```python
from build123d import *

# Parameters (mm, degrees)
SKETCH1_R           = 3.38
SKETCH1_W           = 189.625170906
SKETCH1_H           = 189.625170906
BOSS_EXTRUDE1_DEPTH = 9.525


with BuildPart() as part:
    # Sketch1 → Boss-Extrude1 (new body)
    with BuildSketch(Plane.XY):
        Polygon((16.997849507, 0), (0, -16.997849507), (0, -195.854150493), (16.997849507, -212.852), (195.854150493, -212.852), (212.852, -195.854150493), (212.852, -16.997849507), (195.854150493, 0), align=None)
        with Locations(Location((30.226, -208.026, 0), (0, 0, 180))):
            Circle(SKETCH1_R, mode=Mode.SUBTRACT)
        with Locations(Location((4.826, -182.626, 0), (0, 0, 180))):
            Circle(SKETCH1_R, mode=Mode.SUBTRACT)
        with Locations(Location((55.626, -208.026, 0), (0, 0, 180))):
            Circle(SKETCH1_R, mode=Mode.SUBTRACT)
        with Locations(Location((81.026, -208.026, 0), (0, 0, 180))):
            Circle(SKETCH1_R, mode=Mode.SUBTRACT)
        with Locations(Location((4.826, -157.226, 0), (0, 0, 180))):
            Circle(SKETCH1_R, mode=Mode.SUBTRACT)
        with Locations(Location((4.826, -131.826, 0), (0, 0, 180))):
            Circle(SKETCH1_R, mode=Mode.SUBTRACT)
        with Locations(Location((4.826, -106.426, 0), (0, 0, 180))):
            Circle(SKETCH1_R, mode=Mode.SUBTRACT)
        with Locations(Location((106.426, -208.026, 0), (0, 0, 180))):
            Circle(SKETCH1_R, mode=Mode.SUBTRACT)
        with Locations(Location((131.826, -208.026, 0), (0, 0, 180))):
            Circle(SKETCH1_R, mode=Mode.SUBTRACT)
        with Locations(Location((157.226, -208.026, 0), (0, 0, 180))):
            Circle(SKETCH1_R, mode=Mode.SUBTRACT)
        with Locations(Location((182.626, -208.026, 0), (0, 0, 180))):
            Circle(SKETCH1_R, mode=Mode.SUBTRACT)
        with Locations(Location((208.026, -182.626, 0), (0, 0, 180))):
            Circle(SKETCH1_R, mode=Mode.SUBTRACT)
        with Locations(Location((208.026, -157.226, 0), (0, 0, 180))):
            Circle(SKETCH1_R, mode=Mode.SUBTRACT)
        with Locations(Location((208.026, -131.826, 0), (0, 0, 180))):
            Circle(SKETCH1_R, mode=Mode.SUBTRACT)
        with Locations(Location((4.826, -81.026, 0), (0, 0, 180))):
            Circle(SKETCH1_R, mode=Mode.SUBTRACT)
        with Locations(Location((4.826, -55.626, 0), (0, 0, 180))):
            Circle(SKETCH1_R, mode=Mode.SUBTRACT)
        with Locations(Location((4.826, -30.226, 0), (0, 0, 180))):
            Circle(SKETCH1_R, mode=Mode.SUBTRACT)
        with Locations(Location((30.226, -4.826, 0), (0, 0, 180))):
            Circle(SKETCH1_R, mode=Mode.SUBTRACT)
        with Locations(Location((55.626, -4.826, 0), (0, 0, 180))):
            Circle(SKETCH1_R, mode=Mode.SUBTRACT)
        with Locations(Location((81.026, -4.826, 0), (0, 0, 180))):
            Circle(SKETCH1_R, mode=Mode.SUBTRACT)
        with Locations((106.426, -106.426)):
            Rectangle(SKETCH1_W, SKETCH1_H, mode=Mode.SUBTRACT)
        with Locations(Location((208.026, -106.426, 0), (0, 0, 180))):
            Circle(SKETCH1_R, mode=Mode.SUBTRACT)
        with Locations(Location((208.026, -81.026, 0), (0, 0, 180))):
            Circle(SKETCH1_R, mode=Mode.SUBTRACT)
        with Locations(Location((208.026, -55.626, 0), (0, 0, 180))):
            Circle(SKETCH1_R, mode=Mode.SUBTRACT)
        with Locations(Location((106.426, -4.826, 0), (0, 0, 180))):
            Circle(SKETCH1_R, mode=Mode.SUBTRACT)
        with Locations(Location((131.826, -4.826, 0), (0, 0, 180))):
            Circle(SKETCH1_R, mode=Mode.SUBTRACT)
        with Locations(Location((157.226, -4.826, 0), (0, 0, 180))):
            Circle(SKETCH1_R, mode=Mode.SUBTRACT)
        with Locations(Location((208.026, -30.226, 0), (0, 0, 180))):
            Circle(SKETCH1_R, mode=Mode.SUBTRACT)
        with Locations(Location((182.626, -4.826, 0), (0, 0, 180))):
            Circle(SKETCH1_R, mode=Mode.SUBTRACT)
    extrude(amount=BOSS_EXTRUDE1_DEPTH)


solid = part.part
```
Can you work these out from the model? Positions are in its coordinate system, mm. A direction names the side the tool comes from. Round coordinates to 2 decimals unless told otherwise and drop trailing zeros. Loops run counter-clockwise (first coordinate to the right, second up) from the corner with the lowest first, then second, coordinate; pieces in that order, holes last.
Item 1: Will these pins go through, and if not, where does the flat tip stop? pin 1 Ø6 at (x, y) = (55.626, -208.026) entering from -Z; pin 2 Ø8 at (x, y) = (55.626, -4.826) entering from -Z.
Item 2: Suppose I cut it at C-C, the plane z = 4.75. State how many separate pieces and enclosed holes the cut face has, then the cut area to 3 significant figures.
Item 3: Which directions (+Z, -Z, +X, -X, +Y, -Y) give clear straight access to the entire face, cutting with the end or side of a thin tool? Please do faces 1 (the flat face through (11.613, -108, 5)), 2 (the flat face through (212.852, -108, 5)).
Item 4: Suppose I cut it at A-A, the plane y = -174. Write out the boundary of the cut face in (x, z) (3 decimals), then the cut area to 3 significant figures.
Item 5: Please list where these lines run through material, in increasing order: L1, parallel to Y at x = 106, z = 2.5; L2, parallel to Y at x = 60.5, z = 2.25; L3, parallel to X at y = -20, z = 5.5.
Item 6: If we mould it in two halves opening along X, with no side actions, what happens to faces 3 (the flat face through (204.234, -204.472, 4.696)), 4 (the cylindrical face through (5.559, -26.926, 4.696))? For each: +X half, -X half, draft (parallel to the pull), parting line (faces both ways), or undercut.
Item 7: Suppose I cut it at B-B, the plane x = 88.5. Write out the boundary of the cut face in (y, z) (3 decimals).
Reported:
1. pin 1: passes through
1. pin 2: stops at z = 0
2. separate pieces: 1
2. enclosed holes: 29
2. area: 7,770 mm2
3. face 1: +Z, -Z
3. face 2: +Z, -Z, +X, +Y, -Y
4. outline: (0, 0) - (11.613, 0) - (11.613, 9.525) - (0, 9.525) - close; (201.239, 0) - (212.852, 0) - (212.852, 9.525) - (201.239, 9.525) - close
4. area: 221 mm2
5. L1: y = -212.85 to -211.38, -204.67 to -201.24, -11.61 to -8.18, -1.47 to 0
5. L2: y = -212.85 to -201.24, -11.61 to 0
5. L3: x = 0 to 11.61, 201.24 to 212.85
6. face 3: +X half
6. face 4: undercut
7. outline: (-212.852, 0) - (-201.239, 0) - (-201.239, 9.525) - (-212.852, 9.525) - close; (-11.613, 0) - (0, 0) - (0, 9.525) - (-11.613, 9.525) - close
